Design review of the part built by this model. Coordinates are the model's own, in mm. A direction names the side the tool comes from. Give positions to 0.01 mm unless a question says otherwise; leave off trailing zeros. Order: outer loops, then holes, each group sorted by start corner. A loop starts at its lowest first (then second) coordinate and runs counter-clockwise, first axis right, second up. Notation, with made-up numbers: (-38.75, 76.5) -> (4.25, 76.5) arc R22 cw to (4.25, 100.5) -> close; hole circle Ø9 at (6, -11.5). An arc over 180 degrees is marked (long way). Return JSON: item names as keys, results as strings.
```python
from build123d import *

# Parameters (mm, degrees)
EXTRUDE1_DEPTH = 9
SKETCH2_W      = 3
SKETCH2_H      = 16.95
EXTRUDE2_DEPTH = 3


with BuildPart() as part:
    # Sketch1 → Extrude1 (new body)
    with BuildSketch(Plane.XY):
        with BuildLine():
            Line((7.5, 0), (7.5, 16.95))
            Line((7.5, 16.95), (-7.5, 16.95))
            Line((-7.5, 16.95), (-7.5, 0))
            ThreePointArc((-7.5, 0), (0, 7.5), (7.5, 0))
        make_face()
    extrude(amount=EXTRUDE1_DEPTH)

    # Sketch2 → Extrude2 (add)
    with BuildSketch(Plane(origin=(7.5, 0, 0), x_dir=(0, 0, -1), z_dir=(1, 0, 0))):
        with Locations((-4.5, 8.475)):
            Rectangle(SKETCH2_W, SKETCH2_H)
    extrude2 = extrude(amount=EXTRUDE2_DEPTH)

    # Mirror1: Extrude2 across plane
    add(extrude2.mirror(Plane.ZY))


solid = part.part
```
Item 1: Machinability: for faces 4 (the face through (7.5, 8, 1)), 5 (the face through (-9, 8, 6)), 6 (the face through (9, 8, 6)), which of the approach directions +Z, -Z, +X, -X, +Y, -Y give a long, thin tool a straight path to every point of the face, cutting with its end or side? Answer none if there is none.
Result set:
{"face 4": "-Z, +X, +Y, -Y", "face 5": "+Z, -X, +Y, -Y", "face 6": "+Z, +X, +Y, -Y"}
Item 2: Wall thickness on L1, parallel to Y at x = 4.5, z = 2.5; L2, parallel to X at y = 15.75, z = 2.5; L3, parallel to X at y = 3.25, z = 1.5: over which ranges is each line inside the solid? List them lowest first. Write a range as [from, to].
Result set:
{"L1": "y = [6, 16.95]", "L2": "x = [-7.5, 7.5]", "L3": "x = [-7.5, -6.76], [6.76, 7.5]"}
Item 3: For pin 1 (1.5 mm diameter, centred on y = 7, z = 8, fed in from +X); pin 2 (1.5 mm diameter, centred on y = 3, z = 8, fed in from -X); pin 3 (0.9 mm diameter, centred on x = -9, y = 9.5, fed in from +Z), all flat-tipped, find the tip position at first contact; note any pin that passes through.
Result set:
{"pin 1": "stops at x = 7.5", "pin 2": "stops at x = -7.5", "pin 3": "stops at z = 6"}
Item 4: Add section C-C (x = 0). Give the boundary of the cut face in (y, z), plus the area to 4 significant figures.
Result set:
{"outline": "(7.5, 0) -> (16.95, 0) -> (16.95, 9) -> (7.5, 9) -> close", "area": "85.05 mm^2"}
Item 5: Mouldability with a two-part tool opening along X and no side actions: class faces 1 (the face through (7.5, 8, 7)), 2 (the face through (-0.16, 7.5, 4.44)), 3 (the face through (9, 0, 5)) as released by +X, released by -X, zero draft, split by the parting line, or undercut.
Result set:
{"face 1": "released by +X", "face 2": "undercut", "face 3": "zero draft"}
Item 6: Add section D-D (z = 5.5). Give the boundary of the cut face in (x, y).
Result set:
{"outline": "(-10.5, 0) -> (-7.5, 0) arc R7.5 cw to (7.5, 0) -> (10.5, 0) -> (10.5, 16.95) -> (-10.5, 16.95) -> close"}
Item 7: Add section A-A (y = 2.5). Give the boundary of the cut face in (x, z).
Result set:
{"outline": "(-10.5, 3) -> (-7.5, 3) -> (-7.5, 0) -> (-7.07, 0) -> (-7.07, 9) -> (-7.5, 9) -> (-7.5, 6) -> (-10.5, 6) -> close; (7.07, 0) -> (7.5, 0) -> (7.5, 3) -> (10.5, 3) -> (10.5, 6) -> (7.5, 6) -> (7.5, 9) -> (7.07, 9) -> close"}
Item 8: Add section B-B (y = 9.75). Give the boundary of the cut face in (x, z), plus the area to 3 significant figures.
Result set:
{"outline": "(-10.5, 3) -> (-7.5, 3) -> (-7.5, 0) -> (7.5, 0) -> (7.5, 3) -> (10.5, 3) -> (10.5, 6) -> (7.5, 6) -> (7.5, 9) -> (-7.5, 9) -> (-7.5, 6) -> (-10.5, 6) -> close", "area": "153 mm^2"}
